from build123d import *

# Parameters (mm, degrees)
SKIZZE3_R                       = 1.6
AUFSATZ_LINEAR_AUSTRAGEN2_DEPTH = 3


with BuildPart() as part:
    # Skizze3 → Aufsatz-Linear austragen2 (new body)
    with BuildSketch(Plane(origin=(0, 0, 0), x_dir=(1, 0, 0), z_dir=(0, 1, 0))):
        with BuildLine():
            Line((-22.920228343, 96.629088178), (-22.344299626, 93.816420414))
            ThreePointArc((-22.344299626, 93.816420414), (-22.542717442, 92.719074618), (-23.44364655, 92.061910889))
            ThreePointArc((-23.44364655, 92.061910889), (-54.271856221, 77.97156932), (-78.191055718, 53.955155506))
            ThreePointArc((-78.191055718, 53.955155506), (-79.120725207, 53.338399316), (-80.219076246, 53.534099474))
            Line((-80.219076246, 53.534099474), (-89.501191513, 59.319472491))
            ThreePointArc((-89.501191513, 59.319472491), (-90.633712755, 59.507661551), (-91.567595966, 58.839917861))
            Line((-91.567595966, 58.839917861), (-93.154445785, 56.293958781))
            ThreePointArc((-93.154445785, 56.293958781), (-93.342634844, 55.161437539), (-92.674891154, 54.22755433))
            Line((-92.674891154, 54.22755433), (-83.39277588, 48.44218132))
            ThreePointArc((-83.39277588, 48.44218132), (-82.733338177, 47.542283842), (-82.877606996, 46.436001751))
            ThreePointArc((-82.877606996, 46.436001751), (-93.904857786, 14.383243174), (-92.977009936, -19.500656997))
            ThreePointArc((-92.977009936, -19.500656997), (-93.170481392, -20.599402805), (-94.069039172, -21.260664834))
            Line((-94.069039172, -21.260664834), (-112.45901324, -26.02283492))
            ThreePointArc((-112.45901324, -26.02283492), (-113.375668635, -26.714038487), (-113.535087151, -27.850966463))
            Line((-113.535087151, -27.850966463), (-112.78302952, -30.755171917))
            ThreePointArc((-112.78302952, -30.755171917), (-112.091825953, -31.671827312), (-110.954897977, -31.831245829))
            Line((-110.954897977, -31.831245829), (-92.56492391, -27.069075743))
            ThreePointArc((-92.56492391, -27.069075743), (-91.458351408, -27.211099875), (-90.755907088, -28.077844089))
            ThreePointArc((-90.755907088, -28.077844089), (-75.123446485, -58.150389407), (-49.929025507, -80.821361112))
            ThreePointArc((-49.929025507, -80.821361112), (-49.266012044, -81.71862735), (-49.405877469, -82.825474774))
            Line((-49.405877469, -82.825474774), (-62.541801916, -106.490431951))
            ThreePointArc((-62.541801916, -106.490431951), (-62.672436625, -107.631025681), (-61.958287752, -108.529919931))
            Line((-61.958287752, -108.529919931), (-59.335285607, -109.985893746))
            ThreePointArc((-59.335285607, -109.985893746), (-58.194691877, -110.116528455), (-57.295797627, -109.402379582))
            Line((-57.295797627, -109.402379582), (-44.159873181, -85.737422405))
            ThreePointArc((-44.159873181, -85.737422405), (-43.294500776, -85.033288783), (-42.182335236, -85.121387406))
            ThreePointArc((-42.182335236, -85.121387406), (18.550993294, -93.171136345), (71.569296393, -62.47268054))
            ThreePointArc((71.569296393, -62.47268054), (71.9321762, -61.340716002), (71.357484514, -60.300160894))
            Line((71.357484514, -60.300160894), (68.971387619, -58.452957067))
            ThreePointArc((68.971387619, -58.452957067), (68.257042933, -52.841387619), (73.868612381, -52.127042933))
            Line((73.868612381, -52.127042933), (76.254709276, -53.97424676))
            ThreePointArc((76.254709276, -53.97424676), (77.40605957, -54.269912054), (78.411007457, -53.635006381))
            ThreePointArc((78.411007457, -53.635006381), (81.195601848, -49.318092427), (83.742774792, -44.856969025))
            add(Edge.make_bspline(
                [(83.742774792, -44.856969025), (85.080044201, -42.885733183), (86.342723056, -40.864226462), (90.475393107, -33.658708882), (92.941125683, -28.24523113), (96.845107593, -17.06419167), (98.283381771, -11.296742285), (100.106464604, 0.398106312), (100.491415891, 6.325362035), (100.215805302, 18.151824424), (99.555347906, 24.050820899), (97.228067455, 35.64317623), (95.561517803, 41.336299316), (91.289247265, 52.354443321), (88.683550867, 57.679431674), (82.621810162, 67.817630372), (79.16582226, 72.63078095), (73.343896748, 79.470957727), (71.24767403, 81.729158793), (69.059455254, 83.893875883)],
                knots=[0.068742517, 0.068742517, 0.068742517, 0.068742517, 0.0703125, 0.0703125, 0.07421875, 0.07421875, 0.078125, 0.078125, 0.08203125, 0.08203125, 0.0859375, 0.0859375, 0.08984375, 0.08984375, 0.09375, 0.09375, 0.09765625, 0.09765625, 0.099693464, 0.099693464, 0.099693464, 0.099693464], degree=3))
            ThreePointArc((69.059455254, 83.893875883), (67.867659856, 84.321246531), (66.773383158, 83.684394547))
            ThreePointArc((66.773383158, 83.684394547), (59.654132804, 78.863219836), (51.13982414, 80.060716878))
            ThreePointArc((51.13982414, 80.060716878), (19.451120952, 92.98738567), (-14.761966333, 93.846067312))
            ThreePointArc((-14.761966333, 93.846067312), (-15.84949093, 94.09499262), (-16.464348853, 95.025918661))
            Line((-16.464348853, 95.025918661), (-17.041794218, 97.835985787))
            ThreePointArc((-17.041794218, 97.835985787), (-17.68563769, 98.786504104), (-18.813021723, 99.003355966))
            Line((-18.813021723, 99.003355966), (-21.752647244, 98.399287425))
            ThreePointArc((-21.752647244, 98.399287425), (-22.702876664, 97.75588212), (-22.920228343, 96.629088178))
        make_face()
        with Locations(Location((-84.889727457, 11.033320997, 0), (0, 0, 270))):
            Circle(SKIZZE3_R, mode=Mode.SUBTRACT)
        with Locations(Location((32.889727457, 79.033320997, 0), (0, 0, 270))):
            Circle(SKIZZE3_R, mode=Mode.SUBTRACT)
        with Locations(Location((84.889727457, -11.033320997, 0), (0, 0, 270))):
            Circle(SKIZZE3_R, mode=Mode.SUBTRACT)
        with Locations(Location((-32.889727457, -79.033320997, 0), (0, 0, 270))):
            Circle(SKIZZE3_R, mode=Mode.SUBTRACT)
        with Locations(Location((97.25, 14.9, 0), (0, 0, 270))):
            Circle(SKIZZE3_R, mode=Mode.SUBTRACT)
        with Locations(Location((8.32, -81.84, 0), (0, 0, 270))):
            Circle(SKIZZE3_R, mode=Mode.SUBTRACT)
        with Locations(Location((-42, 40, 0), (0, 0, 270))):
            Circle(SKIZZE3_R, mode=Mode.SUBTRACT)
        with Locations(Location((0, 55.75, 0), (0, 0, 270))):
            Circle(SKIZZE3_R, mode=Mode.SUBTRACT)
        with Locations(Location((-45.965517241, 44.163793104, 0), (0, 0, 270))):
            Circle(SKIZZE3_R, mode=Mode.SUBTRACT)
        with Locations(Location((-52.075687148, -60.652605619, 0), (0, 0, 270))):
            Circle(SKIZZE3_R, mode=Mode.SUBTRACT)
        with Locations(Location((8.901557721, -87.560514891, 0), (0, 0, 270))):
            Circle(SKIZZE3_R, mode=Mode.SUBTRACT)
        with BuildLine():
            Line((-1.595893079, 49.88543439), (-78.291651246, 5.605117767))
            ThreePointArc((-78.291651246, 5.605117767), (-79.689428725, 3.78349869), (-79.389727457, 1.507041555))
            Line((-79.389727457, 1.507041555), (-76.889727457, -2.823085464))
            ThreePointArc((-76.889727457, -2.823085464), (-76.789827035, -3.581904509), (-77.255752861, -4.189110868))
            ThreePointArc((-77.255752861, -4.189110868), (-77.721678687, -4.796317226), (-77.621778265, -5.555136271))
            Line((-77.621778265, -5.555136271), (-49.129993275, -54.904355472))
            ThreePointArc((-49.129993275, -54.904355472), (-49.715633921, -57.089996118), (-47.529993275, -57.675636764))
            Line((-47.529993275, -57.675636764), (-43.621778265, -64.444863729))
            ThreePointArc((-43.621778265, -64.444863729), (-43.014571906, -64.910789555), (-42.255752861, -64.810889132))
            ThreePointArc((-42.255752861, -64.810889132), (-41.496933816, -64.71098871), (-40.889727457, -65.176914536))
            Line((-40.889727457, -65.176914536), (-38.389727457, -69.507041555))
            ThreePointArc((-38.389727457, -69.507041555), (-36.568108381, -70.904819034), (-34.291651246, -70.605117767))
            Line((-34.291651246, -70.605117767), (78.291651246, -5.605117767))
            ThreePointArc((78.291651246, -5.605117767), (79.689428725, -3.78349869), (79.389727457, -1.507041555))
            Line((79.389727457, -1.507041555), (76.889727457, 2.823085464))
            ThreePointArc((76.889727457, 2.823085464), (76.789827035, 3.581904509), (77.255752861, 4.189110868))
            ThreePointArc((77.255752861, 4.189110868), (77.721678687, 4.796317226), (77.621778265, 5.555136271))
            Line((77.621778265, 5.555136271), (43.621778265, 64.444863729))
            ThreePointArc((43.621778265, 64.444863729), (43.014571906, 64.910789555), (42.255752861, 64.810889132))
            ThreePointArc((42.255752861, 64.810889132), (41.496933816, 64.71098871), (40.889727457, 65.176914536))
            Line((40.889727457, 65.176914536), (38.389727457, 69.507041555))
            ThreePointArc((38.389727457, 69.507041555), (36.568108381, 70.904819034), (34.291651246, 70.605117767))
            Line((34.291651246, 70.605117767), (0.897163269, 51.324801143))
            ThreePointArc((0.897163269, 51.324801143), (-0.8, 51.385640646), (-1.595893079, 49.88543439))
        make_face(mode=Mode.SUBTRACT)
    extrude(amount=AUFSATZ_LINEAR_AUSTRAGEN2_DEPTH)


solid = part.part
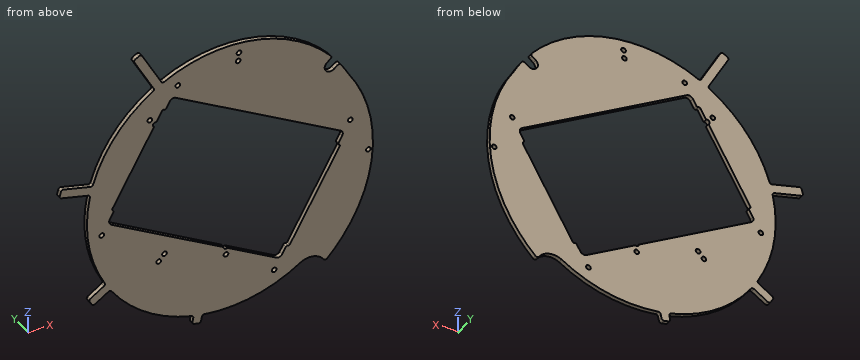
Part model, mm, in its own coordinate system. Round coordinates to 2 decimals unless told otherwise and drop trailing zeros. Return JSON: item names as keys, results as strings. Group by question number.
(1) Pin check, flat tip, straight feed: pin 1 Ø3 at (x, z) = (-84.89, -11.03) entering from -Y. Stop position of the tip, or through.
(2) Drill centre lines: probe 1 along Z at (x, y) = (-34, 1.35); probe 2 along X at (y, z) = (1.25, -14); probe 3 along Z at (x, y) = (-59, 1.85). Where is each one in solid material? Low to high.
(3) Saw through at A-A on y = 1.9. Count the separate pieces of the cut face and the enclosed holes in it, then the cut area to 3 significant figures.
Returned:
{
 "1": {"pin 1": "through"},
 "2": {"probe 1": "-88.71 to -31.18, 70.44 to 77.88, 80.19 to 88.71", "probe 2": "-93.96 to -63.75, 72.75 to 95.93, 98.57 to 100.3", "probe 3": "-74.46 to -16.74, 37.81 to 74.46, 100.11 to 110.12"},
 "3": {"separate pieces": "1", "enclosed holes": "12", "area": "17,400 mm²"}
}
